Job drawing, mm, ordinate dimensions from the low corner. One solid piece. Round coordinates to 2 decimals unless told otherwise and drop trailing zeros. Loops run counter-clockwise (first coordinate to the right, second up) from the corner with the lowest first, then second, coordinate; pieces in that order, holes last. Notation, with made-up numbers: M 52.25,-36 L 56.25,-36 A20 ccw 56.25,-23 Z; hole C 34,-8.75 d2. An arc over 180 degrees is marked long. Write each question's results on one line, items separated by ' | '. Start each with the question number.
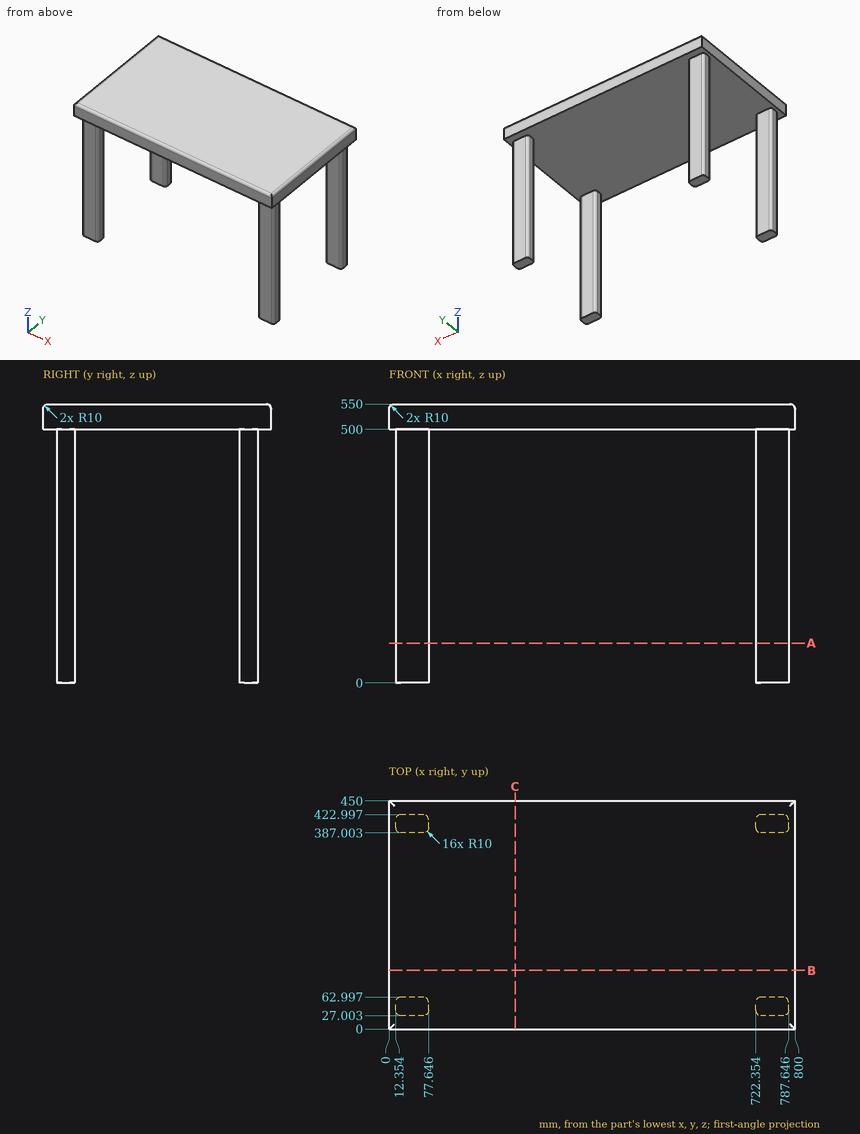
Item 1: Saw through at C-C, the plane x = 248. Give the cut face in (y, z), then the cut area to 3 significant figures.
Item 2: Drill centre lines: line 1 along Y through (x, z) = (71, 403.5); line 2 along Z through (x, y) = (39, 341); line 3 along Y through (x, z) = (74, 171). Where is each one in solid material? Low to high. Write a range as [from, to].
Item 3: Drop flat-ended pins along their axis: pin 1 (13 mm diameter, centred on y = 46.5, z = 237.5, fed in from -X); pin 2 (17.5 mm diameter, centred on y = 404.5, z = 220, fed in from +X); pin 3 (10 mm diameter, centred on x = 300.5, y = 313.5, fed in from -Z). Give the stop position or say it passes through.
Item 4: Saw through at A-A, the plane z = 78.5. State how many separate pieces and enclosed holes the cut face has, then the cut area to 3 significant figures.
Item 5: Saw through at B-B, the plane y = 116. Give the cut face in (x, z), then the cut area to 3 significant figures.
Working result:
1) outline: M 0,500 L 450,500 L 450,540 A10 ccw 440,550 L 10,550 A10 ccw 0,540 Z | area: 22,500 mm²
2) line 1: y = [27.58, 62.42], [387.58, 422.42] | line 2: z = [500, 550] | line 3: y = [29.28, 60.72], [389.28, 420.72]
3) pin 1: stops at x = 12.35 | pin 2: stops at x = 787.65 | pin 3: stops at z = 500
4) separate pieces: 4 | enclosed holes: 0 | area: 9,060 mm²
5) outline: M 0,500 L 800,500 L 800,540 A10 ccw 790,550 L 10,550 A10 ccw 0,540 Z | area: 40,000 mm²
